Input: part model. Units: mm. Frame: model coordinates. A direction names the side the tool comes from. Coordinates: 2 decimals unless noted, no trailing zeros. Write each loop counter-clockwise with the first axis right and the second up, starting at its lowest first coordinate (ties: lowest second). Pieces come first, ordered by that corner, then holes. Notation, with made-up numbers: (78, 40.25) - (94, 40.25) arc R22 cw to (94, 52.25) - close; hole circle Ø8 at (-6, 39). An arc over 180 degrees is marked (long way). Use CSV: the item, a comma, the result in double quotes.
```python
from build123d import *

# Parameters (mm, degrees)
RESSALTO_EXTRUS_O1_DEPTH = 20
RESSALTO_EXTRUS_O2_START = -11.5
RESSALTO_EXTRUS_O2_DEPTH = 14.5
ESBO_O4_R                = 3.5
ESBO_O4_R_2              = 3
RESSALTO_EXTRUS_O3_DEPTH = 11.5


with BuildPart() as part:
    # Esboço1 → Revolução1 (revolve)
    with BuildSketch(Plane.XY):
        Polygon((0, 52.008683422), (0, -22.491316578), (1.15, -22.491316578), (1.15, -21.491316578), (5, -21.491316578), (5, -18.991316578), (13.75, -18.991316578), (13.75, -5.591316578), (14.5, -5.591316578), (14.5, 14.208683422), (17, 14.208683422), (17, 40.208683422), (16.75, 40.208683422), (16.75, 41.508683422), (17, 41.508683422), (17, 52.008683422), align=None)
    revolve(axis=Axis((0, 52.008683422, 0), (0, -1, 0)))

    # Esboço2 → Ressalto-extrusão1 (add)
    with BuildSketch(Plane(origin=(0, 52.008683422, 0), x_dir=(1, 0, 0), z_dir=(0, 1, 0))):
        with BuildLine():
            Line((15.092560694, 11.367260519), (16.033467531, 12.075923108))
            ThreePointArc((16.033467531, 12.075923108), (21.020085445, 10.947420147), (19.086085546, 6.214606868))
            Line((19.086085546, 6.214606868), (17.966039096, 5.849909332))
            ThreePointArc((17.966039096, 5.849909332), (16.852954176, 4.947741706), (16.628916094, 3.532583974))
            Line((16.628916094, 3.532583974), (9.846019669, 0))
            Line((9.846019669, 0), (16.628916094, -3.532583974))
            ThreePointArc((16.628916094, -3.532583974), (16.852954176, -4.947741706), (17.966039096, -5.849909332))
            Line((17.966039096, -5.849909332), (19.086085546, -6.214606868))
            ThreePointArc((19.086085546, -6.214606868), (21.020085445, -10.947420147), (16.033467531, -12.075923108))
            Line((16.033467531, -12.075923108), (15.092560694, -11.367260519))
            ThreePointArc((15.092560694, -11.367260519), (13.715258298, -10.972415516), (12.427288325, -11.600107969))
            Line((12.427288325, -11.600107969), (0, -5.127881824))
            Line((0, -5.127881824), (-12.427288325, -11.600107969))
            ThreePointArc((-12.427288325, -11.600107969), (-13.715258298, -10.972415516), (-15.092560694, -11.367260519))
            Line((-15.092560694, -11.367260519), (-16.033467531, -12.075923108))
            ThreePointArc((-16.033467531, -12.075923108), (-21.020085445, -10.947420147), (-19.086085546, -6.214606868))
            Line((-19.086085546, -6.214606868), (-17.966039096, -5.849909332))
            ThreePointArc((-17.966039096, -5.849909332), (-16.852954176, -4.947741706), (-16.628916094, -3.532583974))
            Line((-16.628916094, -3.532583974), (-9.846019669, 0))
            Line((-9.846019669, 0), (-16.628916094, 3.532583974))
            ThreePointArc((-16.628916094, 3.532583974), (-16.852954176, 4.947741706), (-17.966039096, 5.849909332))
            Line((-17.966039096, 5.849909332), (-19.086085546, 6.214606868))
            ThreePointArc((-19.086085546, 6.214606868), (-21.020085445, 10.947420147), (-16.033467531, 12.075923108))
            Line((-16.033467531, 12.075923108), (-15.092560694, 11.367260519))
            ThreePointArc((-15.092560694, 11.367260519), (-13.715258298, 10.972415516), (-12.427288325, 11.600107969))
            Line((-12.427288325, 11.600107969), (0, 5.127881824))
            Line((0, 5.127881824), (12.427288325, 11.600107969))
            ThreePointArc((12.427288325, 11.600107969), (13.715258298, 10.972415516), (15.092560694, 11.367260519))
        make_face()
    extrude(amount=-RESSALTO_EXTRUS_O1_DEPTH)

    # Esboço3 → Ressalto-extrusão2 (add)
    with BuildSketch(Plane(origin=(0, 52.008683422, 0), x_dir=(1, 0, 0), z_dir=(0, 1, 0)).offset(RESSALTO_EXTRUS_O2_START)):
        with BuildLine():
            Line((-20.55, -3.25), (-18.065620285, -3.429043833))
            ThreePointArc((-18.065620285, -3.429043833), (-16.957055718, -3.864486935), (-16.292605909, -4.852936501))
            Line((-16.292605909, -4.852936501), (-16.292605909, 4.852936501))
            ThreePointArc((-16.292605909, 4.852936501), (-16.957055718, 3.864486935), (-18.065620285, 3.429043833))
            Line((-18.065620285, 3.429043833), (-20.55, 3.25))
            ThreePointArc((-20.55, 3.25), (-23.8, 0), (-20.55, -3.25))
        make_face()
        with BuildLine():
            Line((16.292605909, -4.852936501), (16.292605909, 4.852936501))
            ThreePointArc((16.292605909, 4.852936501), (16.957055718, 3.864486935), (18.065620285, 3.429043833))
            Line((18.065620285, 3.429043833), (20.55, 3.25))
            ThreePointArc((20.55, 3.25), (23.8, 0), (20.55, -3.25))
            Line((20.55, -3.25), (18.065620285, -3.429043833))
            ThreePointArc((18.065620285, -3.429043833), (16.957055718, -3.864486935), (16.292605909, -4.852936501))
        make_face()
    extrude(amount=-RESSALTO_EXTRUS_O2_DEPTH)

    # Esboço4 → Ressalto-extrusão3 (add)
    with BuildSketch(Plane(origin=(0, 52.008683422, 0), x_dir=(1, 0, 0), z_dir=(0, 1, 0))):
        with Locations((0, -9.25)):
            Circle(ESBO_O4_R)
        with Locations((0, -9.25)):
            Circle(ESBO_O4_R_2, mode=Mode.SUBTRACT)
        with Locations((0, 9.25)):
            Circle(ESBO_O4_R)
        with Locations((0, 9.25)):
            Circle(ESBO_O4_R_2, mode=Mode.SUBTRACT)
    extrude(amount=RESSALTO_EXTRUS_O3_DEPTH)


solid = part.part
```
(1) Ray query, probe 1 along Z at (x, y) = (0, 60); probe 2 along X at (y, z) = (61.25, -9.25); probe 3 along Y at (x, z) = (6.5, -14.5). Return the intervals inside material, ascending. Write a range as from..to.
Check values:
probe 1,"-12.75..-12.25, -6.25..-5.75, 5.75..6.25, 12.25..12.75"
probe 2,"-3.5..-3, 3..3.5"
probe 3,"14.21..52.01"
(2) Pin query (flat end, axial travel): pin 1 Ø6 at (x, z) = (-19, -0.5) entering from -Y; pin 2 Ø5 at (y, z) = (3, 0.5) entering from -X; pin 3 Ø1.5 at (y, z) = (26.5, 1) entering from +X. Return the tip coordinate at first contact, or that it passes through.
Check values:
pin 1,"y = 14.21"
pin 2,"x = -14.5"
pin 3,"x = 23.79"
(3) Draft query along Z for faces 1 (the cylindrical face through (0.19, 40.87, 16.75)), 2 (the flat face through (0, 52.009, 9)), 3 (the cylindrical face through (-2.981, -12.198, -13.423)). Return one class per face: pulls with the +Z half, pulls with the -Z half, needs draft (parallel to the pull), parting line crosses it, or undercut.
Check values:
face 1,"pulls with the +Z half"
face 2,"undercut"
face 3,"parting line crosses it"
(4) Cut plane C-C on y = -17. Return loops of the section in (x, z).
Check values:
outline,"circle Ø27.5 at (0, 0)"
(5) Cut plane A-A on y = 53. Return loops of the section in (x, z).
Check values:
outline,"circle Ø7 at (0, -9.25); circle Ø7 at (0, 9.25); hole circle Ø6 at (0, -9.25); hole circle Ø6 at (0, 9.25)"
(6) Reachability of faces 4 (the cylindrical face through (17, 47, 0)), 5 (the flat face through (-18, 32.009, -9)), 6 (the cylindrical face through (-16.863, 42.149, 4.965)) from +Z, -Z, +X, -X, +Y, -Y: full face, straight path, thin tool, end or side. Return the list, or none.
Check values:
face 4,"+X, +Y"
face 5,"-Z, -X, -Y"
face 6,"-X, +Y"
(7) Cut plane D-D on z = -9.25. Return loops of the section in (x, y).
Check values:
outline,"(-21.4, 32.01) - (-14.26, 32.01) - (-14.26, 14.21) - (-11.17, 14.21) - (-11.17, -5.59) - (-10.17, -5.59) - (-10.17, -18.99) - (10.17, -18.99) - (10.17, -5.59) - (11.17, -5.59) - (11.17, 14.21) - (14.26, 14.21) - (14.26, 32.01) - (21.4, 32.01) - (21.4, 52.01) - (3.5, 52.01) - (3.5, 63.51) - (3, 63.51) - (3, 52.01) - (-3, 52.01) - (-3, 63.51) - (-3.5, 63.51) - (-3.5, 52.01) - (-21.4, 52.01) - close"
